Verification items for the finished model (mm, model axes). Face numbers are marked on the shaded views. A direction names the side the tool comes from. Coordinates: 2 decimals unless noted, no trailing zeros. Loops run counter-clockwise (first coordinate to the right, second up) from the corner with the lowest first, then second, coordinate; pieces in that order, holes last.
Q1. Sectioned sample at C-C (x = 4). Enter the section's corners in (y, z).
Q2. Access from +Z, -Z, +X, -X, +Y, -Y to the whole of each face (thin tool, end or side, straight path). Record for the marked faces 4, 5 and 6.
Q3. Material ranges on probe 1 along X at (y, z) = (-65.5, 27); probe 2 along X at (y, z) = (-72.5, 12.75); probe 3 along Z at (x, y) = (14.5, -125.5), recorded low to high.
Q4. Sectioned sample at B-B (y = -120). Enter the section's corners in (x, z).
Q5. Sectioned sample at A-A (z = 15.25). Enter the section's corners in (x, y), then the cut area to 3 significant figures.
Q6. Go/stop test with flat-tipped pins: P1, Ø0.5, axis at x = -11, y = -63, coming from the +Z side; P2, Ø2, axis at y = -80.5, z = 26.5, coming from the -X side; P3, Ø6, axis at x = 11, z = 22, coming from the -Y side. Record where each tip stops, or that it passes through.
Q7. Mould release check, pull along X, two halves, no side actions. Record for the marked faces 1, 2 and 3: +X half, -X half, draft (parallel to the pull), parting line (faces both ways), or undercut.
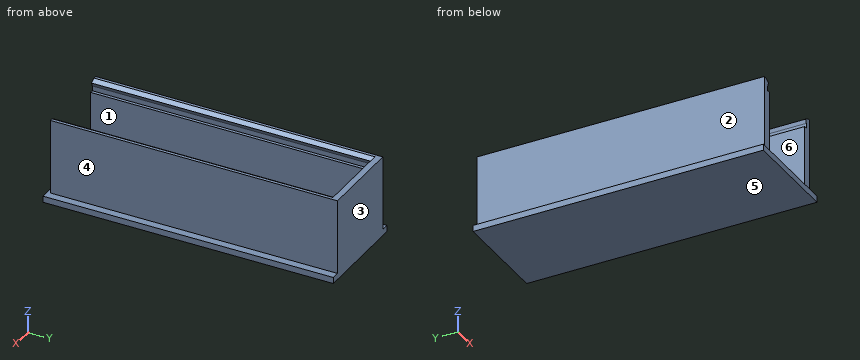
```python
from build123d import *

# Parameters (mm, degrees)
SKETCH010_W  = 32
SKETCH010_H  = 93
PAD008_DEPTH = 2
PAD009_DEPTH = 90
SKETCH012_W  = 27
SKETCH012_H  = 2
PAD010_DEPTH = 3
PAD011_DEPTH = 24


with BuildPart() as part:
    # Sketch010 → Pad008 (new body)
    with BuildSketch(Plane.XY):
        with Locations((0, -84.5)):
            Rectangle(SKETCH010_W, SKETCH010_H)
    extrude(amount=PAD008_DEPTH)

    # Sketch011 → Pad009 (join)
    with BuildSketch(Plane.XZ.offset(40)):
        Polygon((-13.5, 2), (-13.5, 26), (-12.5, 26), (-11.085595, 25.117329), (-11.5, 23.95), (-11.5, 22.35), (-10.5, 22.35), (-10.5, 2), align=None)
    pad009 = extrude(amount=PAD009_DEPTH)

    # Mirrored: Pad009 across Sketch011 V_Axis
    add(pad009.mirror(Plane(origin=(0, -40, 0), x_dir=(0, -1, 0), z_dir=(1, 0, 0))))

    # Sketch012 (on Face5 of Mirrored) → Pad010 (join)
    with BuildSketch(Plane.XY.offset(2)):
        with Locations((0, -39)):
            Rectangle(SKETCH012_W, SKETCH012_H)
    extrude(amount=PAD010_DEPTH)

    # Sketch012 (on Face5 of Mirrored) → Pad011 (join)
    with BuildSketch(Plane.XY.offset(2)):
        with Locations((0, -39)):
            Rectangle(SKETCH012_W, SKETCH012_H)
    extrude(amount=PAD011_DEPTH)


with BuildPart() as part_1:
    # Body006 placement: moved
    add(part.part.moved(Location((0, 0, 4))))


solid = part_1.part
```
Geometry check:
1. outline: (-131, 4) - (-38, 4) - (-38, 30) - (-40, 30) - (-40, 6) - (-131, 6) - close
2. face 4: +Z, +X, +Y, -Y
2. face 5: -Z, +X, -X, +Y, -Y
2. face 6: +Z, -Y
3. probe 1: x = -13.5 to -11.5, 11.5 to 13.5
3. probe 2: x = -13.5 to -10.5, 10.5 to 13.5
3. probe 3: z = 4 to 6
4. outline: (-16, 4) - (16, 4) - (16, 6) - (13.5, 6) - (13.5, 30) - (12.5, 30) - (11.09, 29.12) - (11.5, 27.95) - (11.5, 26.35) - (10.5, 26.35) - (10.5, 6) - (-10.5, 6) - (-10.5, 26.35) - (-11.5, 26.35) - (-11.5, 27.95) - (-11.09, 29.12) - (-12.5, 30) - (-13.5, 30) - (-13.5, 6) - (-16, 6) - close
5. outline: (-13.5, -130) - (-10.5, -130) - (-10.5, -40) - (10.5, -40) - (10.5, -130) - (13.5, -130) - (13.5, -38) - (-13.5, -38) - close
5. area: 594 mm2
6. P1: stops at z = 29.22
6. P2: stops at x = -13.5
6. P3: stops at y = -130
7. face 1: undercut
7. face 2: -X half
7. face 3: draft
